Work out the finished part from the listing and answer in its coordinate system (mm). A direction names the side the tool comes from. Coordinates: 2 decimals unless noted, no trailing zeros. Order: outer loops, then holes, each group sorted by start corner. A loop starts at its lowest first (then second) coordinate and runs counter-clockwise, first axis right, second up. Notation, with made-up numbers: (28, 37.5) -> (65, 37.5) arc R30 ccw to (65, 59.5) -> close; hole circle Ø11 at (41, 61.5). An arc over 180 degrees is marked (long way). Write item = value, one per line. Start each with the question number.
Q1. The part is cut by section D-D, the plane x = 20. Determine the outline of the cut face in (y, z), plus the area to 3 significant figures.
Q2. Which of the six approach directions +Z, -Z, +X, -X, +Y, -Y give full straight-line access (tool end or side, diameter ignored) to faces 5 (the flat face through (3, 9, 0)), 6 (the cylindrical face through (-9.76, 133.6, -2.17)), 7 (the flat face through (-7, 235, 0)), 8 (the flat face through (-3, 9, 0))?
Q3. Straight lines are drawn through the part: L1, parallel to X at y = 173, z = 0; L2, parallel to X at y = 65.5, z = 0; L3, parallel to Y at x = -12, z = 16. For each, find the intervals that lie inside material, in ascending order. Write a range as from..to.
Q4. The part is cut by section A-A, the plane y = 102.5. Determine the outline of the cut face in (x, z), plus the area to 3 significant figures.
Q5. Flat-ended cylindrical pins translate along their axes: pin 1 (10 mm diameter, centred on x = 21, z = 23, fed in from -Y); pin 2 (2 mm diameter, centred on y = 8, z = -0.5, fed in from +X); pin 3 (5.5 mm diameter, centred on y = 7.5, z = 0, fed in from -X). Find the tip coordinate at first contact, or state that the pin passes through.
Q6. The part is cut by section B-B, the plane y = 49.5. Determine the outline of the cut face in (x, z), plus the area to 3 significant figures.
Q7. For a pull along X with two mould halves and no side action, classify faces 1 (the cylindrical face through (1.802, 18.123, 5.723)), 2 (the cylindrical face through (1.802, 153.88, 5.723)), 3 (the flat face through (1, 30, 8)), 4 (the flat face through (0, 75, 0)) as +X half, -X half, draft (parallel to the pull), parting line (faces both ways), or undercut.
Q8. The part is cut by section C-C, the plane z = -13. Determine the outline of the cut face in (x, y), plus the area to 3 significant figures.
```python
from build123d import *

# Parameters (mm, degrees)
SCHIZZO1_R                   = 6
ESTRUSIONE_ESTRUSIONE1_DEPTH = 30
SCHIZZO2_R                   = 40
ESTRUSIONE_ESTRUSIONE2_DEPTH = 5
SCHIZZO3_R                   = 10
ESTRUSIONE_ESTRUSIONE3_DEPTH = 200
TAGLIO_ESTRUSIONE1_START     = -160
SCHIZZO4_R                   = 6
TAGLIO_ESTRUSIONE1_DEPTH     = 160
SCHIZZO5_W                   = 3
SCHIZZO5_H                   = 13
TAGLIO_ESTRUSIONE2_DEPTH     = 242.712639305
RACCORDO1_R                  = 3


with BuildPart() as part:
    # Schizzo1 → Estrusione-Estrusione1 (new body)
    with BuildSketch(Plane(origin=(0, 0, 0), x_dir=(1, 0, 0), z_dir=(0, 1, 0))):
        with Locations(Location((0, 0, 0), (0, 0, 270))):
            Circle(SCHIZZO1_R)
    extrude(amount=ESTRUSIONE_ESTRUSIONE1_DEPTH)

    # Schizzo2 → Estrusione-Estrusione2 (add)
    with BuildSketch(Plane(origin=(0, 30, 0), x_dir=(1, 0, 0), z_dir=(0, 1, 0))):
        with Locations(Location((0, 0, 0), (0, 0, 270))):
            Circle(SCHIZZO2_R)
    extrude(amount=ESTRUSIONE_ESTRUSIONE2_DEPTH)

    # Schizzo3 → Estrusione-Estrusione3 (add)
    with BuildSketch(Plane(origin=(0, 35, 0), x_dir=(1, 0, 0), z_dir=(0, 1, 0))):
        with Locations(Location((0, 0, 0), (0, 0, 270))):
            Circle(SCHIZZO3_R)
    extrude(amount=ESTRUSIONE_ESTRUSIONE3_DEPTH)

    # Schizzo4 → Taglio-Estrusione1 (cut)
    with BuildSketch(Plane(origin=(0, 235, 0), x_dir=(1, 0, 0), z_dir=(0, 1, 0)).offset(TAGLIO_ESTRUSIONE1_START)):
        with Locations(Location((0, 0, 0), (0, 0, 270))):
            Circle(SCHIZZO4_R)
    extrude(amount=TAGLIO_ESTRUSIONE1_DEPTH, mode=Mode.SUBTRACT)

    # Schizzo5 → Taglio-Estrusione2 (cut, symmetric)
    with BuildSketch(Plane.XY):
        with Locations((4.5, 6.5)):
            Rectangle(SCHIZZO5_W, SCHIZZO5_H)
    taglio_estrusione2 = extrude(amount=TAGLIO_ESTRUSIONE2_DEPTH, both=True, mode=Mode.SUBTRACT)

    # Specchia1: Taglio-Estrusione2 across plane
    add(taglio_estrusione2.mirror(Plane(origin=(0, 0, 0), x_dir=(0, 0, 1), z_dir=(1, 0, 0))), mode=Mode.SUBTRACT)


with BuildPart() as body_2:
    # Schizzo6 → Rivoluzione1 (revolve)
    with BuildSketch(Plane(origin=(0, 0, 0), x_dir=(0, 0, -1), z_dir=(1, 0, 0))):
        with BuildLine():
            Line((-4, 6.058790505), (4, 6.058790505))
            ThreePointArc((4, 6.058790505), (0, 10.058790505), (-4, 6.058790505))
        make_face()
    revolve(axis=Axis((0, 6.058790505, 4), (0, 0, -1)))


with BuildPart() as part_1:
    add(part.part)

    # Abbina1: cut body 2
    add(body_2.part, mode=Mode.SUBTRACT)

    # Raccordo1
    raccordo1_edges = [part_1.edges().sort_by_distance(p)[0] for p in [
        (3, 0, 0),
        (-3, 0, 0),
        (-3, 13, 0),
        (3, 13, 0),
    ]]
    fillet(raccordo1_edges, radius=RACCORDO1_R - 0.0001)  # a hair under: the kernel refuses the full size


solid = part_1.part
```
Model answer:
q1.outline = (30, -34.64) -> (35, -34.64) -> (35, 34.64) -> (30, 34.64) -> close
q1.area = 346 mm2
q2.face_5 = +Z, -Z, +X, -Y
q2.face_6 = +Y
q2.face_7 = +Z, -Z, +X, -X, +Y
q2.face_8 = +Z, -Z, -X, -Y
q3.L1 = -10..-6, 6..10
q3.L2 = -10..10
q3.L3 = 30..35
q4.outline = circle Ø20 at (0, 0); hole circle Ø12 at (0, 0)
q4.area = 201 mm2
q5.pin_1 = 30
q5.pin_2 = 3
q5.pin_3 = -3.01
q6.outline = circle Ø20 at (0, 0)
q6.area = 314 mm2
q7.face_1 = parting line
q7.face_2 = undercut
q7.face_3 = draft
q7.face_4 = undercut
q8.outline = (-37.83, 30) -> (37.83, 30) -> (37.83, 35) -> (-37.83, 35) -> close
q8.area = 378 mm2
